For this review, use the dimensioned drawing (mm, ordinates from the lowest corner) and the shaded views. A direction names the side the tool comes from. Give positions to 0.01 mm unless a question says otherwise; leave off trailing zeros. Loops run counter-clockwise (first coordinate to the right, second up) from the corner with the lowest first, then second, coordinate; pieces in that order, holes last. Notation, with made-up numbers: (43, 27.25) - (83, 27.25) arc R17 cw to (83, 45.25) - close; hole circle Ø4 at (-11.75, 72). An arc over 180 degrees is marked (long way). Write each question's results on one line, items separated by ' | '.
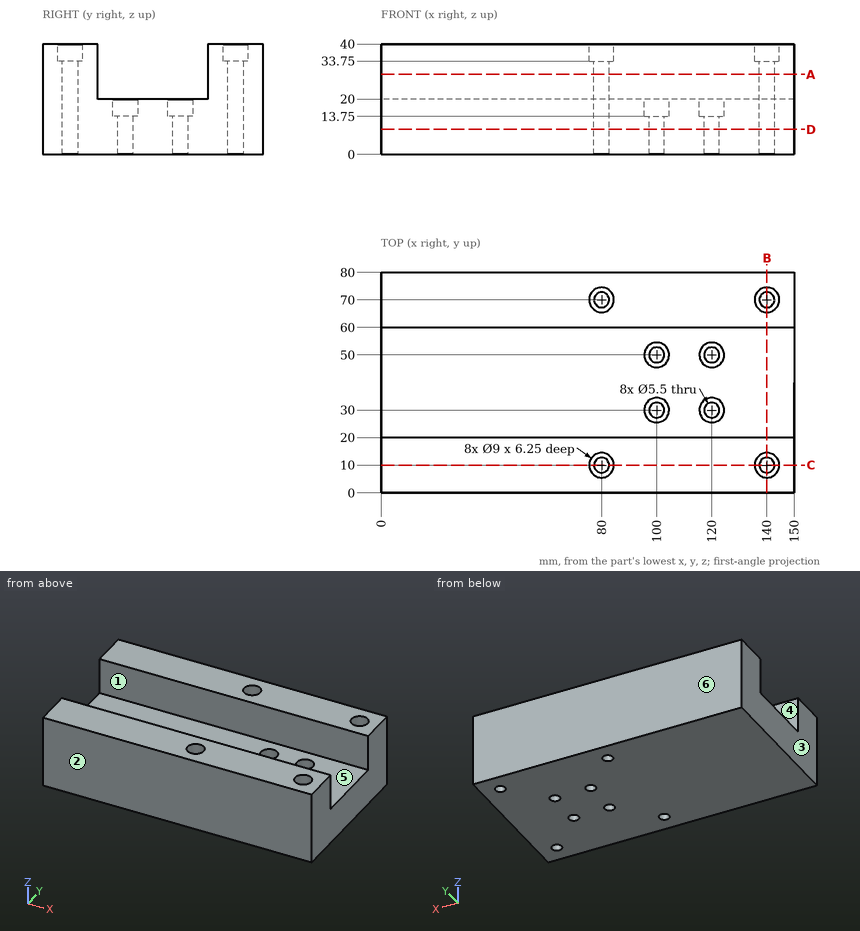
Item 1: Tool access review of the marked faces 5 and 6: name each direction out of +Z, -Z, +X, -X, +Y, -Y from which nothing blocks a thin tool from reaching the whole face with its end or side.
Output values:
face 5: +Z, +X, -X | face 6: +Z, -Z, +X, -X, +Y
Item 2: Clearance check with flat-ended pins moving along their axes: P1, Ø8, axis at x = 100, y = 50, coming from the +Z side; P2, Ø4.5, axis at x = 140, y = 70, coming from the -Z side; P3, Ø2.5, axis at x = 80.5, y = 11.5, coming from the +Z side; P4, Ø12, axis at x = 62.5, y = 33, coming from the +Z side. State where each tip first meets the part, or that it passes through.
Output values:
P1: stops at z = 13.75 | P2: passes through | P3: stops at z = 33.75 | P4: stops at z = 20
Item 3: Draft analysis for pull direction Y (two halves, no side actions). For the marked faces 1, 2, 3 and 4, state which applies: +Y half, -Y half, draft (parallel to the pull), parting line (faces both ways), or undercut.
Output values:
face 1: undercut | face 2: -Y half | face 3: draft | face 4: undercut
Item 4: We need section C-C on y = 10. Give the boundary of the cut face in (x, z), then the cut area to 3 significant figures.
Output values:
outline: (0, 0) - (77.25, 0) - (77.25, 33.75) - (75.5, 33.75) - (75.5, 40) - (0, 40) - close; (82.75, 0) - (137.25, 0) - (137.25, 33.75) - (135.5, 33.75) - (135.5, 40) - (84.5, 40) - (84.5, 33.75) - (82.75, 33.75) - close; (142.75, 0) - (150, 0) - (150, 40) - (144.5, 40) - (144.5, 33.75) - (142.75, 33.75) - close | area: 5,520 mm²
Item 5: We need section A-A on z = 29. Give the boundary of the cut face in (x, y).
Output values:
outline: (0, 0) - (150, 0) - (150, 20) - (0, 20) - close; (0, 60) - (150, 60) - (150, 80) - (0, 80) - close; hole circle Ø5.5 at (80, 10); hole circle Ø5.5 at (80, 70); hole circle Ø5.5 at (140, 10); hole circle Ø5.5 at (140, 70)
Item 6: We need section B-B on x = 140. Give the boundary of the cut face in (y, z), then the cut area to 3 significant figures.
Output values:
outline: (0, 0) - (7.25, 0) - (7.25, 33.75) - (5.5, 33.75) - (5.5, 40) - (0, 40) - close; (12.75, 0) - (67.25, 0) - (67.25, 33.75) - (65.5, 33.75) - (65.5, 40) - (60, 40) - (60, 20) - (20, 20) - (20, 40) - (14.5, 40) - (14.5, 33.75) - (12.75, 33.75) - close; (72.75, 0) - (80, 0) - (80, 40) - (74.5, 40) - (74.5, 33.75) - (72.75, 33.75) - close | area: 1,920 mm²
Item 7: We need section D-D on z = 9. Give the number of separate pieces and of enclosed holes in the cut face, then the cut area to 3 significant figures.
Output values:
separate pieces: 1 | enclosed holes: 8 | area: 11,800 mm²
Item 8: Wall thickness on probe 1 along Y at (x, z) = (100, 6.75); probe 2 along Y at (x, z) = (100, 19.5); probe 3 along X at (y, z) = (50, 17): over which ranges is each line inside the solid? List them lowest first.
Output values:
probe 1: y = 0 to 27.25, 32.75 to 47.25, 52.75 to 80 | probe 2: y = 0 to 25.5, 34.5 to 45.5, 54.5 to 80 | probe 3: x = 0 to 95.5, 104.5 to 115.5, 124.5 to 150
